```python
from build123d import *

# Parameters (mm, degrees)
F0_W     = 31.851116
F0_H     = 31.851116
F1_DEPTH = 31
F2_R     = 5.164209
F3_DEPTH = 3
F4_R     = 4.113364
F4_R_2   = 3.901474
F5_DEPTH = 3


with BuildPart() as f1:
    # F0 (on Top) → F1 (new body)
    with BuildSketch(Plane.XY):
        Rectangle(F0_W, F0_H)
    extrude(amount=F1_DEPTH)

    # F2 (on face) → F3 (cut)
    with BuildSketch(Plane.XY.offset(31)):
        with Locations((-8.903265, 7.398488)):
            Circle(F2_R)
        with Locations((8.903265, 7.398488)):
            Circle(F2_R)
        with Locations((8.903265, -7.398488)):
            Circle(F2_R)
        with Locations((-8.903265, -7.398488)):
            Circle(F2_R)
    extrude(amount=-F3_DEPTH, mode=Mode.SUBTRACT)

    # F4 (on face) → F5 (cut)
    with BuildSketch(Plane(origin=(0, 0, 0), x_dir=(1, 0, 0), z_dir=(0, 0, -1))):
        with Locations((-9.906449, 9.655653)):
            Circle(F4_R)
        Circle(F4_R)
        with Locations((9.404857, -10.408042)):
            Circle(F4_R_2)
    extrude(amount=-F5_DEPTH, mode=Mode.SUBTRACT)


solid = f1.part
```
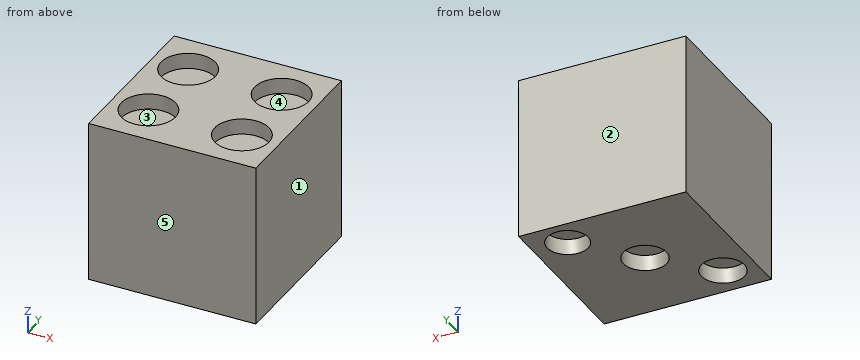
For this review, take the finished solid that the model builds, in its own axes (mm). Face numbers are marked on the shaded views. A direction names the side the tool comes from. Round coordinates to 2 decimals unless told otherwise and drop trailing zeros. Write each loop counter-clockwise with the first axis right and the second up, starting at its lowest first coordinate (ties: lowest second). Pieces come first, ordered by that corner, then holes. Notation, with made-up numbers: (70.25, 11.5) -> (112.25, 11.5) arc R13 cw to (112.25, 18.5) -> close; hole circle Ø1 at (-19.75, 87). An arc over 180 degrees is marked (long way). One line per question, with ' | ' between items. Start each with the question number.
(1) For line 1 along Y through (x, z) = (5, 30); line 2 along Y through (x, z) = (7.5, 29); line 3 along Z through (x, y) = (-4.5, 10), list the stretches that pass through material, from the lowest coordinate up. Write a range as from..to.
(2) Add section A-A, the plane y = 0. Write out the cut boundary in (x, z), plus the area to 3 significant figures.
(3) Mouldability with a two-part tool opening along Y and no side actions: class the marked faces 1, 2 and 3 as released by +Y, released by -Y, zero draft, split by the parting line, or undercut.
(4) Add section C-C, the plane x = 10. Write out the cut boundary in (y, z), plus the area to 3 significant figures.
(5) Insertion check: P1, Ø11.5, axis at x = 8.5, y = -9.5, coming from the +Z side; P2, Ø6, axis at x = -8.9, y = 7.4, coming from the +Z side. Each pin has a flat end and moves straight along its axis. Give the tip position at first contact, or say it passes through.
(6) Tool access review of the marked faces 4 and 5: name each direction out of +Z, -Z, +X, -X, +Y, -Y from which nothing blocks a thin tool from reaching the whole face with its end or side.
Answer list:
1) line 1: -15.93..-10.78, -4.02..4.02, 10.78..15.93 | line 2: -15.93..-12.37, -2.43..2.43, 12.37..15.93 | line 3: 0..28
2) outline: (-15.93, 0) -> (-4.11, 0) -> (-4.11, 3) -> (4.11, 3) -> (4.11, 0) -> (15.93, 0) -> (15.93, 31) -> (-15.93, 31) -> close | area: 963 mm²
3) face 1: zero draft | face 2: released by +Y | face 3: undercut
4) outline: (-15.93, 0) -> (6.55, 0) -> (6.55, 3) -> (14.26, 3) -> (14.26, 0) -> (15.93, 0) -> (15.93, 31) -> (12.44, 31) -> (12.44, 28) -> (2.35, 28) -> (2.35, 31) -> (-2.35, 31) -> (-2.35, 28) -> (-12.44, 28) -> (-12.44, 31) -> (-15.93, 31) -> close | area: 904 mm²
5) P1: z = 31 | P2: z = 28
6) face 4: +Z | face 5: +Z, -Z, +X, -X, -Y
